For this review, take the finished solid that the model builds, in its own axes (mm). Coordinates: 2 decimals unless noted, no trailing zeros. Order: outer loops, then holes, each group sorted by start corner. A loop starts at its lowest first (then second) coordinate and runs counter-clockwise, first axis right, second up. Notation, with made-up numbers: (-32.5, 66) - (-26.5, 66) arc R13 ccw to (-26.5, 73) - close; hole circle Ø1 at (-3.5, -35.75). An arc over 180 degrees is marked (long way). One line per item, written item: value. Start each with the question number.
(1) Consider section A-A on x = -2.5. Write out the cut boundary in (y, z).
(2) Consider section B-B on y = 1.7. Count the separate pieces of the cut face and the enclosed holes in it, then the cut area to 3 significant figures.
(3) To check wall thickness, follow line 1 along Z through (x, y) = (-2.5, 1.85); line 2 along Z through (x, y) = (43.5, 2.6); line 3 along X through (y, z) = (0.95, -5). State the ranges of each line that lie inside material, in increasing order.
(4) Consider section C-C on x = 45. Write out the cut boundary in (y, z).
(5) Clearance check with flat-ended pins moving along their axes: pin 1 (5 mm diameter, centred on x = 45.5, z = -4, fed in from +Y); pin 2 (0.9 mm diameter, centred on x = -21, y = 1.5, fed in from -Z); pin 3 (0.9 mm diameter, centred on y = 1.5, z = -16, fed in from -X); pin 4 (0.9 mm diameter, centred on x = 28, y = 1.5, fed in from +Z). State where each tip first meets the part, or that it passes through.
(6) Consider section D-D on z = -13.5. Write out the cut boundary in (x, y), then the cut area to 3 significant figures.
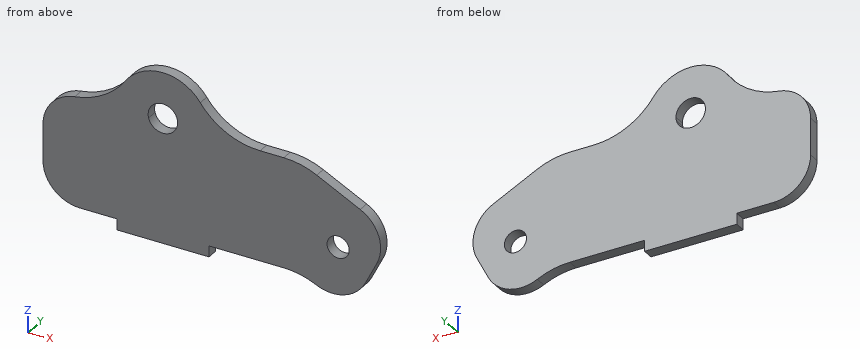
```python
from build123d import *

# Parameters (mm, degrees)
SKETCH1_R           = 3
SKETCH1_W           = 25
SKETCH1_H           = 3
BOSS_EXTRUDE1_DEPTH = 3
FILLET1_R           = 10
FILLET2_R           = 20


with BuildPart() as part:
    # Sketch1 → Boss-Extrude1 (new body)
    with BuildSketch(Plane(origin=(0, 0, 0), x_dir=(1, 0, 0), z_dir=(0, 1, 0))):
        with BuildLine():
            Line((10, -16), (10, -15))
            Line((10, -15), (1.372983346, -15))
            ThreePointArc((1.372983346, -15), (1.468118785, -15.49598283), (1.5, -16))
            ThreePointArc((1.5, -16), (-3.00401717, -19.968118785), (-6.372983346, -15))
            Line((-6.372983346, -15), (-15, -15))
            Line((-15, -15), (-15, -16))
            ThreePointArc((-15, -16), (-2.5, -28.5), (10, -16))
        make_face()
        with BuildLine():
            Line((47.94427191, 21.472135955), (35, 15))
            Line((35, 15), (10, 15))
            Line((10, 15), (10, 12))
            Line((10, 12), (-15, 12))
            Line((-15, 12), (-15, 15))
            Line((-15, 15), (-35, 15))
            Line((-35, 15), (-35, -15))
            Line((-35, -15), (-15, -15))
            Line((-15, -15), (-6.372983346, -15))
            ThreePointArc((-6.372983346, -15), (-2.5, -12), (1.372983346, -15))
            Line((1.372983346, -15), (10, -15))
            Line((10, -15), (35, -15))
            Line((35, -15), (59.94427191, -2.527864045))
            Line((59.94427191, -2.527864045), (47.94427191, 21.472135955))
        make_face()
        with Locations((45, 5)):
            Circle(SKETCH1_R, mode=Mode.SUBTRACT)
        with Locations((-2.5, 16.5)):
            Rectangle(SKETCH1_W, SKETCH1_H)
        with Locations((-2.5, 13.5)):
            Rectangle(SKETCH1_W, SKETCH1_H)
    extrude(amount=BOSS_EXTRUDE1_DEPTH)

    # Fillet1
    fillet1_edges = [part.edges().sort_by_distance(p)[0] for p in [
        (47.94427191, 1.5, -21.472135955),
        (59.94427191, 1.5, 2.527864045),
        (-35, 1.5, 15),
        (-35, 1.5, -15),
    ]]
    fillet(fillet1_edges, radius=FILLET1_R)

    # Fillet2
    fillet2_edges = [part.edges().sort_by_distance(p)[0] for p in [
        (35, 1.5, -15),
        (35, 1.5, 15),
        (10, 1.5, 15),
        (-15, 1.5, 15),
    ]]
    fillet(fillet2_edges, radius=FILLET2_R)


solid = part.part
```
Geometry check:
1. outline: (0, -18) - (3, -18) - (3, 12) - (0, 12) - close; (0, 20) - (3, 20) - (3, 28.5) - (0, 28.5) - close
2. separate pieces: 1
2. enclosed holes: 2
2. area: 2,900 mm^2
3. line 1: z = -18 to 12, 20 to 28.5
3. line 2: z = -18.06 to -7.6, -2.4 to 10.75
3. line 3: x = -35 to 42, 48 to 56.05
4. outline: (0, -17.94) - (3, -17.94) - (3, -8) - (0, -8) - close; (0, -2) - (3, -2) - (3, 10) - (0, 10) - close
5. pin 1: stops at y = 3
5. pin 2: stops at z = -15
5. pin 3: stops at x = -15
5. pin 4: stops at z = 15
6. outline: (-30.27, 0) - (51.86, 0) - (51.86, 3) - (-30.27, 3) - close
6. area: 246 mm^2
